```python
from build123d import *

# Parameters (mm, degrees)
SKETCH2_R           = 3.02870098
BOSS_EXTRUDE1_DEPTH = 14
SKETCH3_W           = 22.225
SKETCH3_H           = 4
SKETCH4_R           = 3.175
CUT_EXTRUDE1_DEPTH  = 4


with BuildPart() as part:
    # Sketch2 → Boss-Extrude1 (new body)
    with BuildSketch(Plane.XY):
        with BuildLine():
            Line((-9.616125613, -19.05), (9.616125613, -19.05))
            Line((9.616125613, -19.05), (9.616125613, 0))
            ThreePointArc((9.616125613, 0), (0, 9.616125613), (-9.616125613, 0))
            Line((-9.616125613, 0), (-9.616125613, -19.05))
        make_face()
        Circle(SKETCH2_R, mode=Mode.SUBTRACT)
    extrude(amount=BOSS_EXTRUDE1_DEPTH)

    # Sketch3 → Revolve1 (revolve)
    with BuildSketch(Plane(origin=(0, 0, 0), x_dir=(0, 0, -1), z_dir=(1, 0, 0))):
        with Locations((4.1125, -21.05)):
            Rectangle(SKETCH3_W, SKETCH3_H)
    revolve(axis=Axis((0, -23.05, 7), (0, 1, 0)))

    # Sketch4 → Cut-Extrude1 (cut)
    with BuildSketch(Plane(origin=(0, -23.05, 0), x_dir=(-1, 0, 0), z_dir=(0, -1, 0))):
        with Locations((0, -7)):
            Circle(SKETCH4_R)
    extrude(amount=-CUT_EXTRUDE1_DEPTH, mode=Mode.SUBTRACT)


solid = part.part
```
Build history of the part. All positions in model axes, mm. A direction names the side the tool comes from. Round coordinates to 2 decimals unless told otherwise and drop trailing zeros. Loops run counter-clockwise (first coordinate to the right, second up) from the corner with the lowest first, then second, coordinate; pieces in that order, holes last. Notation, with made-up numbers: M 37.5,63 L 89.5,63 A6 ccw 89.5,69 Z; hole C 89.25,86.25 d10. An arc over 180 degrees is marked long. Answer as CSV lines item,"result".
1. Two-plate mould, pull along Y, no slides. Class faces 6 (the cylindrical face through (-0.657, -2.957, 6.902)), 7 (the flat face through (5, -23.05, 7)), 8 (the cylindrical face through (0.211, 9.614, 6.902)), 9 (the flat face through (0, -5, 14)): released by +Y, released by -Y, zero draft, split by the parting line, or undercut.
Resolved:
face 6,"undercut"
face 7,"released by -Y"
face 8,"released by +Y"
face 9,"zero draft"
2. Cut at B-B on y = -1.5. Write the cut outline in (x, z), then the cut area to 3 significant figures.
Resolved:
outline,"M -9.62,0 L -2.63,0 L -2.63,14 L -9.62,14 Z; M 2.63,0 L 9.62,0 L 9.62,14 L 2.63,14 Z"
area,"196 mm²"
3. Wall check: probe 1 along Z at (x, y) = (0, -21) (3 decimals); probe 2 along Y at (x, z) = (0, 7.5); probe 3 along Y at (x, z) = (-6.5, 26). Give the ranges that are in metal, low to high. Write a range as [from, to].
Resolved:
probe 1,"z = [-15.225, 3.825], [10.175, 29.225]"
probe 2,"y = [-19.05, -3.03], [3.03, 9.62]"
probe 3,"y = [-23.05, -19.05]"
4. Flat gauge pins, fed straight in: P1, Ø10, axis at y = -12.5, z = 15.5, coming from the -X side; P2, Ø5, axis at y = -13.5, z = 14.5, coming from the +X side; P3, Ø5, axis at x = -1.5, z = 8, coming from the -Y side; P4, Ø9.5, axis at x = 1, y = -2.5, coming from the -Z side. Where does each tip first touch, or does it go through?
Resolved:
P1,"stops at x = -9.62"
P2,"stops at x = 9.62"
P3,"stops at y = -23.05"
P4,"stops at z = 0"
5. Cut at C-C on z = 7. Write the cut outline in (x, y) (3 decimals).
Resolved:
outline,"M -22.225,-23.05 L -3.175,-23.05 L -3.175,-19.05 L 3.175,-19.05 L 3.175,-23.05 L 22.225,-23.05 L 22.225,-19.05 L 9.616,-19.05 L 9.616,0 A9.616 ccw -9.616,0 L -9.616,-19.05 L -22.225,-19.05 Z; hole C 0,0 d6.057"
6. Cut at A-A on x = 0. Write the cut outline in (y, z) (3 decimals), then the cut area to 3 significant figures.
Resolved:
outline,"M -23.05,-15.225 L -19.05,-15.225 L -19.05,0 L -3.029,0 L -3.029,14 L -19.05,14 L -19.05,29.225 L -23.05,29.225 L -23.05,10.175 L -19.05,10.175 L -19.05,3.825 L -23.05,3.825 Z; M 3.029,0 L 9.616,0 L 9.616,14 L 3.029,14 Z"
area,"469 mm²"
7. 3-axis set-ups, long thin cutter, end or side, ignore diameter. For faces 1 (the cylindrical face through (-6.676, -21.022, -14.199)), 2 (the cylindrical face through (-1.5, -21.1, 9.8)), 3 (the flat face through (9.616, -10, 7)), 4 (the flat face through (0, -5, 0)), 5 (the flat face through (-9.616, -9, 7)): which of +Z, -Z, +X, -X, +Y, -Y reach the whole face in a straight line?
Resolved:
face 1,"+Y, -Y"
face 2,"-Y"
face 3,"+Z, -Z, +X, +Y"
face 4,"-Z, +X, -X, +Y"
face 5,"+Z, -Z, -X, +Y"
8. Cut at D-D on y = -5. Write the cut outline in (x, z), then the cut area to 3 significant figures.
Resolved:
outline,"M -9.62,0 L 9.62,0 L 9.62,14 L -9.62,14 Z"
area,"269 mm²"
